Design review of the part shown in the three views and the two pictorial views. Dimensions are in mm from the part's minimum x, y and z. Coordinates: 2 decimals unless noted, no trailing zeros. Loops run counter-clockwise (first coordinate to the right, second up) from the corner with the lowest first, then second, coordinate; pieces in that order, holes last. Notation, with made-up numbers: (-31, 46) - (14, 46) arc R16 cw to (14, 70) - close; hole circle Ø4 at (53, 61). An arc over 180 degrees is marked (long way). One line per question, with ' | ' between items.
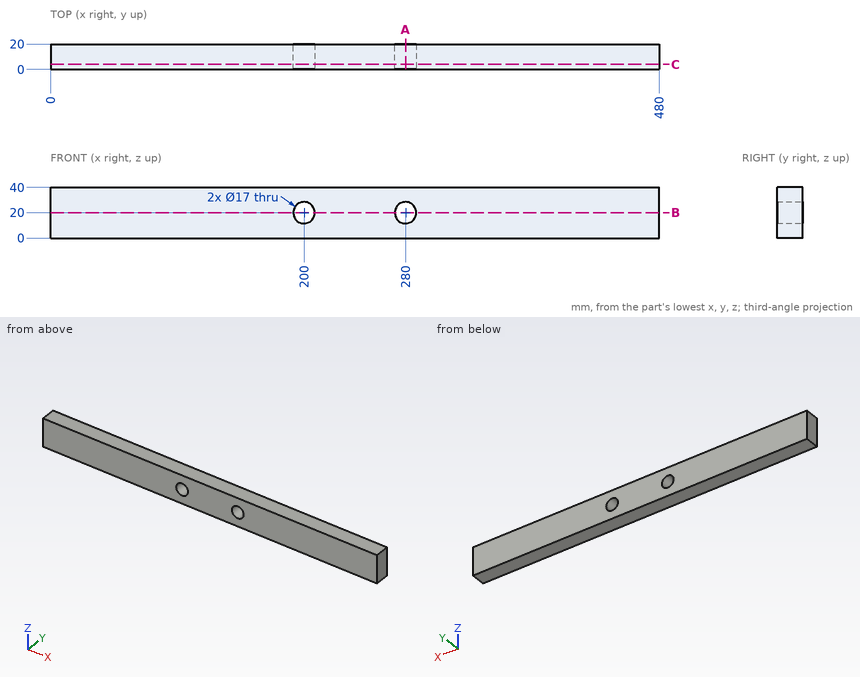
Q1. Take a section at A-A (x = 280). Give the boundary of the cut face in (y, z).
Returned:
outline: (0, 0) - (20, 0) - (20, 11.5) - (0, 11.5) - close; (0, 28.5) - (20, 28.5) - (20, 40) - (0, 40) - close
Q2. Take a section at C-C (y = 4). Give the boundary of the cut face in (x, z), plus the area to 3 significant figures.
Returned:
outline: (0, 0) - (480, 0) - (480, 40) - (0, 40) - close; hole circle Ø17 at (200, 20); hole circle Ø17 at (280, 20) | area: 18,700 mm²
Q3. Take a section at B-B (z = 20). Give the boundary of the cut face in (x, y), plus the area to 3 significant figures.
Returned:
outline: (0, 0) - (191.5, 0) - (191.5, 20) - (0, 20) - close; (208.5, 0) - (271.5, 0) - (271.5, 20) - (208.5, 20) - close; (288.5, 0) - (480, 0) - (480, 20) - (288.5, 20) - close | area: 8,920 mm²
Q4. To check wall thickness, follow line 1 along Z through (x, y) = (200, 7); line 2 along X through (y, z) = (12, 16.5); line 3 along X through (y, z) = (7.5, 22.5). State the ranges of each line that lie inside material, in increasing order.
Returned:
line 1: z = 0 to 11.5, 28.5 to 40 | line 2: x = 0 to 192.25, 207.75 to 272.25, 287.75 to 480 | line 3: x = 0 to 191.88, 208.12 to 271.88, 288.12 to 480
